```python
from build123d import *

# Parameters (mm, degrees)
F3_DEPTH = 14.2


with BuildPart() as f2:
    # F1 (on Front) → F2 (revolve)
    with BuildSketch(Plane.XZ):
        Polygon((-14.2, 40), (-14.2, 0), (14.2, 0), (14.2, 40), (11.2, 40), (8.0834, 27.5), (4.6166, 27.5), (1.5, 40), (-1.5, 40), (-4.6166, 27.5), (-8.0834, 27.5), (-11.2, 40), align=None)
    revolve(axis=Axis((0, 0, 0), (-1, 0, 0)))

    # F0 (on Right) → F3 (cut, symmetric)
    with BuildSketch(Plane.YZ):
        with BuildLine():
            Line((-17.3, -4), (-12.369317, -4))
            ThreePointArc((-12.369317, -4), (13, 0), (-12.369317, 4))
            Line((-12.369317, 4), (-17.3, 4))
            Line((-17.3, 4), (-17.3, -4))
        make_face()
    extrude(amount=F3_DEPTH, both=True, mode=Mode.SUBTRACT)


solid = f2.part
```
Check sheet for the modelled part. Datum: model origin and axes. Units: mm. A direction names the side the tool comes from. Coordinates: 2 decimals unless noted, no trailing zeros. Order: outer loops, then holes, each group sorted by start corner. A loop starts at its lowest first (then second) coordinate and runs counter-clockwise, first axis right, second up. Notation, with made-up numbers: (17, 73) -> (51, 73) arc R22 ccw to (51, 109) -> close; hole circle Ø9 at (51, 28). An arc over 180 degrees is marked (long way). Write each question's results on one line, items separated by ' | '. Start each with the question number.
1) Section check B-B (z = 0). Enter the section's corners in (x, y), and give its area (3 significant figures).
2) Section check C-C (y = -30). Count the separate pieces of the cut face and the enclosed holes in it, and give its area (3 significant figures).
3) Set-up check for faces 1 (the face through (-14.2, 9.4, -9.4)), 2 (the face through (-8.28, -27.61, -6.13)), 3 (the face through (0, -15, 4)): record each of +Z, -Z, +X, -X, +Y, -Y from which the full face is reachable in a straight line by a thin tool's end or side.
4) Draft check along Y on faces 4 (the face through (0.2, 12.99, -0.51)), 5 (the face through (14.2, 9.4, 9.4)), 6 (the face through (0, -15, -4)), 7 (the face through (-0.02, -39.05, -8.67)). Enter one of: pulls with the +Y half, pulls with the -Y half, needs draft (parallel to the pull), parting line crosses it, or undercut.
5) Section check A-A (y = 0). Enter the section's corners in (x, z), and give its area (3 significant figures).
6) Material ranges on line 1 along X through (y, z) = (-28.5, 2.5); line 2 along Y through (x, z) = (6.75, 0); line 3 along Y through (x, z) = (-0.5, 0), recorded low to high.
7) Depth check by flat-ended pin: pin 1 (10 mm diameter, centred on x = -3.5, z = -17, fed in from -Y); pin 2 (4 mm diameter, centred on x = 1.5, y = -14, fed in from +Z); pin 3 (6.5 mm diameter, centred on x = 0.5, z = -0.5, fed in from +Y). Enter the tip coordinate at first touch or a pass-through.
Checked values:
1) outline: (-14.2, -40) -> (-11.2, -40) -> (-8.08, -27.5) -> (-4.62, -27.5) -> (-1.5, -40) -> (1.5, -40) -> (4.62, -27.5) -> (8.08, -27.5) -> (11.2, -40) -> (14.2, -40) -> (14.2, -17.3) -> (-14.2, -17.3) -> close; (-14.2, 13) -> (14.2, 13) -> (14.2, 40) -> (11.2, 40) -> (8.08, 27.5) -> (4.62, 27.5) -> (1.5, 40) -> (-1.5, 40) -> (-4.62, 27.5) -> (-8.08, 27.5) -> (-11.2, 40) -> (-14.2, 40) -> close | area: 1,080 mm²
2) separate pieces: 3 | enclosed holes: 0 | area: 818 mm²
3) face 1: +Z, -Z, -X, +Y, -Y | face 2: none | face 3: +X, -X
4) face 4: undercut | face 5: needs draft | face 6: undercut | face 7: parting line crosses it
5) outline: (-14.2, -40) -> (-11.2, -40) -> (-8.08, -27.5) -> (-4.62, -27.5) -> (-1.5, -40) -> (1.5, -40) -> (4.62, -27.5) -> (8.08, -27.5) -> (11.2, -40) -> (14.2, -40) -> (14.2, -13) -> (-14.2, -13) -> close; (-14.2, 13) -> (14.2, 13) -> (14.2, 40) -> (11.2, 40) -> (8.08, 27.5) -> (4.62, 27.5) -> (1.5, 40) -> (-1.5, 40) -> (-4.62, 27.5) -> (-8.08, 27.5) -> (-11.2, 40) -> (-14.2, 40) -> close | area: 1,200 mm²
6) line 1: -14.2 to -8.36, -4.34 to 4.34, 8.36 to 14.2 | line 2: -27.5 to -17.3, 13 to 27.5 | line 3: -40 to -17.3, 13 to 40
7) pin 1: y = -38.02 | pin 2: z = 38.16 | pin 3: y = 40
